```python
from build123d import *

# Parameters (mm, degrees)
BOSS_EXTRUDE1_DEPTH = 6.35


with BuildPart() as part:
    # Sketch1 → Boss-Extrude1 (new body)
    with BuildSketch(Plane.XY):
        Polygon((0, -6.35), (19.05, -6.35), (19.05, 0), (34.925, 0), (41.275, 0), (41.275, 10.795), (34.925, 10.795), (34.925, 19.07), (31.115, 19.07), (31.115, 17.07), (29.115, 17.07), (29.115, 19.07), (24.765, 19.07), (24.765, 21.57), (29.115, 21.57), (29.115, 23.57), (31.115, 23.57), (31.115, 21.57), (34.925, 21.57), (34.925, 29.845), (41.275, 29.845), (41.275, 60.325), (34.925, 60.325), (26.65, 60.325), (26.65, 56.515), (28.65, 56.515), (28.65, 54.515), (26.65, 54.515), (26.65, 50.165), (24.15, 50.165), (24.15, 54.515), (22.15, 54.515), (22.15, 56.515), (24.15, 56.515), (24.15, 60.325), (19.05, 60.325), (19.05, 66.675), (0, 66.675), (0, 60.325), (-5.1, 60.325), (-5.1, 56.515), (-3.1, 56.515), (-3.1, 54.515), (-5.1, 54.515), (-5.1, 50.165), (-7.6, 50.165), (-7.6, 54.515), (-9.6, 54.515), (-9.6, 56.515), (-7.6, 56.515), (-7.6, 60.325), (-15.875, 60.325), (-22.225, 60.325), (-22.225, 29.845), (-15.875, 29.845), (-15.875, 21.57), (-12.065, 21.57), (-12.065, 23.57), (-10.065, 23.57), (-10.065, 21.57), (-5.715, 21.57), (-5.715, 19.07), (-10.065, 19.07), (-10.065, 17.07), (-12.065, 17.07), (-12.065, 19.07), (-15.875, 19.07), (-15.875, 10.795), (-22.225, 10.795), (-22.225, 0), (-15.875, 0), (0, 0), align=None)
    extrude(amount=BOSS_EXTRUDE1_DEPTH)


solid = part.part
```
For this review, take the finished solid that the model builds, in its own axes (mm). A direction names the side the tool comes from. Coordinates: 2 decimals unless noted, no trailing zeros. Write each loop counter-clockwise with the first axis right and the second up, starting at its lowest first coordinate (ties: lowest second). Pieces come first, ordered by that corner, then holes. Notation, with made-up numbers: (72.25, -19) - (99.25, -19) arc R24 ccw to (99.25, -1) - close; hole circle Ø2 at (50.25, -14). An arc over 180 degrees is marked (long way). Answer in a Markdown table with one row per item. Add a question column.
Q1. We need section B-B, the plane y = 22.5. State the section outline as (x, z) points (3 decimals), and give its area (3 significant figures).
Q2. Tool access review of faces 1 (the flat face through (0, 64, 3)), 2 (the flat face through (30, 17.07, 3)), 3 (the flat face through (-14, 19.07, 3)), 4 (the flat face through (24.15, 52, 3)), 5 (the flat face through (34.925, 26, 3)): name each direction out of +Z, -Z, +X, -X, +Y, -Y from which nothing blocks a thin tool from reaching the whole face with its end or side.
Q3. For probe 1 along X at (y, z) = (18.5, 0.5) (3 decimals); probe 2 along X at (y, z) = (50.5, 1.25) (3 decimals); probe 3 along Y at (x, z) = (29.5, 6) (3 decimals), list the stretches that pass through material, from the lowest coordinate up.
Q4. For P1, Ø1.9, axis at y = 64.5, z = 3.5, coming from the +X side; P2, Ø3, axis at x = 34.5, z = 2.5, coming from the -Y side; P3, Ø3, axis at x = -5, z = 3, coming from the +Y side (3 decimals), all flat-tipped, find the tip position at first contact; note any pin that passes through.
Q5. Draft analysis for pull direction Y (two halves, no side actions). For faces 6 (the flat face through (25, 50.165, 3)), 7 (the flat face through (34.925, 15, 3)), 8 (the flat face through (26.65, 58, 3)), state which applies: +Y half, -Y half, draft (parallel to the pull), parting line (faces both ways), or undercut.
Q6. We need section C-C, the plane x = -8.5. State the section outline as (y, z) points (3 decimals), and give its area (3 significant figures).
Q7. We need section A-A, the plane x = -15. State the section outline as (y, z) points (3 decimals).
Answer list:
| question | item | result |
|---|---|---|
| 1 | outline | (-15.875, 0) - (-12.065, 0) - (-12.065, 6.35) - (-15.875, 6.35) - close; (-10.065, 0) - (29.115, 0) - (29.115, 6.35) - (-10.065, 6.35) - close; (31.115, 0) - (34.925, 0) - (34.925, 6.35) - (31.115, 6.35) - close |
| 1 | area | 297 mm2 |
| 2 | face 1 | +Z, -Z, -X, +Y |
| 2 | face 2 | +Z, -Z |
| 2 | face 3 | +Z, -Z, -X |
| 2 | face 4 | +Z, -Z, +Y |
| 2 | face 5 | +Z, -Z, +X |
| 3 | probe 1 | x = -15.875 to -12.065, -10.065 to 29.115, 31.115 to 34.925 |
| 3 | probe 2 | x = -22.225 to -7.6, -5.1 to 24.15, 26.65 to 41.275 |
| 3 | probe 3 | y = 0 to 17.07, 23.57 to 60.325 |
| 4 | P1 | stops at x = 19.05 |
| 4 | P2 | stops at y = 0 |
| 4 | P3 | stops at y = 60.325 |
| 5 | face 6 | +Y half |
| 5 | face 7 | undercut |
| 5 | face 8 | draft |
| 6 | outline | (0, 0) - (19.07, 0) - (19.07, 6.35) - (0, 6.35) - close; (21.57, 0) - (54.515, 0) - (54.515, 6.35) - (21.57, 6.35) - close; (56.515, 0) - (60.325, 0) - (60.325, 6.35) - (56.515, 6.35) - close |
| 6 | area | 354 mm2 |
| 7 | outline | (0, 0) - (19.07, 0) - (19.07, 6.35) - (0, 6.35) - close; (21.57, 0) - (60.325, 0) - (60.325, 6.35) - (21.57, 6.35) - close |
